Input: part model. Units: mm. Frame: model coordinates. Face numbers are marked on the shaded views. A direction names the side the tool comes from. Round coordinates to 2 decimals unless told otherwise and drop trailing zeros. Loops run counter-clockwise (first coordinate to the right, second up) from the corner with the lowest first, then second, coordinate; pieces in that order, holes last. Notation, with made-up numbers: (-8.75, 68) - (42.25, 68) arc R14 cw to (42.25, 95) - close; hole circle Ø3 at (-25, -14). An arc over 180 degrees is marked (long way). One line per question, with ' | ' between items. Start each with the question number.
Autodesk Inventor part; units mm, degrees
ref_plane "YZ Plane" through (0, 0, 0) normal (1, 0, 0) x (0, 1, 0)
ref_plane "XZ Plane" through (0, 0, 0) normal (0, 1, 0) x (-1, 0, 0)
ref_plane "XY Plane" through (0, 0, 0) normal (0, 0, 1) x (1, 0, 0)
sketch "Sketch1" plane through (0, 0, 0) normal (0, 0, 1) x (1, 0, 0)
  line L0 (-12.1708, 16.0073) -> (13.2292, 16.0073)
  line L1 (13.2292, 16.0073) -> (13.2292, -34.7927)
  line L2 (13.2292, -34.7927) -> (-12.1708, -34.7927)
  line L3 (-12.1708, -34.7927) -> (-12.1708, 16.0073)
  line L4 (11.9592, 14.7373) -> (-10.9008, 14.7373)
  line L5 (-10.9008, 14.7373) -> (-10.9008, -33.5227)
  line L6 (-10.9008, -33.5227) -> (11.9592, -33.5227)
  line L7 (11.9592, -33.5227) -> (11.9592, 14.7373)
  point P0 (0, 0)
  dimension "d0" = 25.4
  dimension "d1" = 50.8
  dimension "d2" = 1.27
extrude "Extrusion1" add sketch "Sketch1" along normal blind 263.906
sketch "Sketch2" plane through (-12.1708, 16.0073, 0) normal (0, 1, 0) x (1, 0, 0)
  circle A0 centre (12.7, -12.7) radius 1.7272
  line L0 (25.4, 0) -> (0, 0)
  line L1 (0, 0) -> (0, -263.906)
  point P0 (12.1708, 0)
  dimension "d5" = 3.4544
  dimension "d6" = 12.7
  dimension "d7" = 12.7
extrude "Extrusion2" cut sketch "Sketch2" against normal through all
pattern_linear "Rectangular Pattern1" count 26 spacing 25.4 along (0, 0, 1) of "Extrusion2"
sketch "Sketch3" plane through (13.2292, -34.7927, 0) normal (1, 0, 0) x (0, 0, -1)
  circle A0 centre (-22.606, 25.4) radius 14.2875
  line L0 (0, 0) -> (0, 50.8)
  line L1 (-263.906, 0) -> (-263.906, 50.8)
  point P0 (0, 34.7927)
  dimension "d15" = 28.575
  dimension "d16" = 22.606
extrude "Extrusion3" cut sketch "Sketch3" against normal through all
equation "\"d3\" = d13"
equation "\"d10\" = d14"
equation "\"d13\" = 263.906"
equation "\"d14\" = d13"
properties part number "VersaFrame 30in"
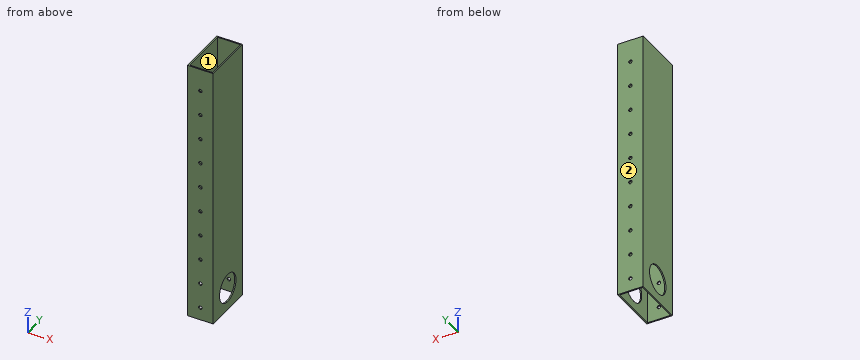
(1) Section A-A, the plane y = 9. Output: boundary loops of the cut face in (x, z), plus the area to 3 significant figures.
(2) Section B-B, the plane z = 23.5. Output: boundary loops of the cut face in (x, y), plus the area to 3 significant figures.
(3) Section C-C, the plane z = 172.5. Output: boundary loops of the cut face in (x, y).
(4) Line query: line 1 along X through (y, z) = (-31.5, 126.5); line 2 along X through (y, z) = (15, 241); line 3 along Y through (x, z) = (9, 146.5). Output: solid intervals per line, ascending. Write a range as from..to.
(5) Reachability of the marked faces 1 and 2 from +Z, -Z, +X, -X, +Y, -Y: full face, straight path, thin tool, end or side. Return the list, or none.
Derived:
1) outline: (-12.17, 0) - (-10.9, 0) - (-10.9, 263.91) - (-12.17, 263.91) - close; (11.96, 0) - (13.23, 0) - (13.23, 263.91) - (11.96, 263.91) - close | area: 670 mm²
2) outline: (-12.17, -34.79) - (13.23, -34.79) - (13.23, -23.65) - (11.96, -23.65) - (11.96, -33.52) - (-10.9, -33.52) - (-10.9, -23.65) - (-12.17, -23.65) - close; (-12.17, 4.87) - (-10.9, 4.87) - (-10.9, 14.74) - (11.96, 14.74) - (11.96, 4.87) - (13.23, 4.87) - (13.23, 16.01) - (-12.17, 16.01) - close | area: 115 mm²
3) outline: (-12.17, -34.79) - (13.23, -34.79) - (13.23, 16.01) - (-12.17, 16.01) - close; hole (-10.9, -33.52) - (11.96, -33.52) - (11.96, 14.74) - (-10.9, 14.74) - close
4) line 1: x = -12.17..-10.9, 11.96..13.23 | line 2: x = -12.17..-1.17, 2.23..13.23 | line 3: y = -34.79..-33.52, 14.74..16.01
5) face 1: +Z, -Z | face 2: +Z, -Z, +X, -X, +Y
